from build123d import *

# Parameters (mm, degrees)
BOSS_EXTRUDE1_DEPTH = 2.5
SKETCH3_R           = 1
CUT_EXTRUDE1_DEPTH  = 5


with BuildPart() as part:
    # Sketch1 → Boss-Extrude1 (new, symmetric)
    with BuildSketch(Plane.XY):
        with BuildLine():
            ThreePointArc((-230.921678322, 34.636363636), (-231.800357978, 32.515043293), (-233.921678322, 31.636363636))
            Line((-233.921678322, 31.636363636), (-233.921678322, 29.636363636))
            ThreePointArc((-233.921678322, 29.636363636), (-233.356489225, 29.668410206), (-232.798545076, 29.764139123))
            ThreePointArc((-232.798545076, 29.764139123), (-230.009155719, 31.52313912), (-228.921678322, 34.636363636))
            Line((-228.921678322, 34.636363636), (-230.921678322, 34.636363636))
        make_face()
        with BuildLine():
            ThreePointArc((-233.921678322, 31.636363636), (-236.042998665, 32.515043293), (-236.921678322, 34.636363636))
            Line((-236.921678322, 34.636363636), (-238.921678322, 34.636363636))
            ThreePointArc((-238.921678322, 34.636363636), (-237.834200924, 31.52313912), (-235.044811567, 29.764139123))
            ThreePointArc((-235.044811567, 29.764139123), (-234.486867419, 29.668410206), (-233.921678322, 29.636363636))
            Line((-233.921678322, 29.636363636), (-233.921678322, 31.636363636))
        make_face()
        with BuildLine():
            ThreePointArc((-232.798545076, 29.764139123), (-233.356489225, 29.668410206), (-233.921678322, 29.636363636))
            Line((-233.921678322, 29.636363636), (-233.921678322, 28.764139123))
            Line((-233.921678322, 28.764139123), (-232.798545076, 28.764139123))
            Line((-232.798545076, 28.764139123), (-232.798545076, 29.764139123))
        make_face()
        with BuildLine():
            ThreePointArc((-233.921678322, 29.636363636), (-234.486867419, 29.668410206), (-235.044811567, 29.764139123))
            Line((-235.044811567, 29.764139123), (-235.044811567, 28.764139123))
            Line((-235.044811567, 28.764139123), (-233.921678322, 28.764139123))
            Line((-233.921678322, 28.764139123), (-233.921678322, 29.636363636))
        make_face()
    extrude(amount=BOSS_EXTRUDE1_DEPTH, both=True)

    # Sketch3 → Cut-Extrude1 (cut)
    with BuildSketch(Plane.XZ.offset(-28.764139123)):
        with Locations(Location((-233.921678322, 0, 0), (0, 0, 270))):
            Circle(SKETCH3_R)
    extrude(amount=-CUT_EXTRUDE1_DEPTH, mode=Mode.SUBTRACT)


solid = part.part
Check sheet for the modelled part. Datum: model origin and axes. Units: mm. Round coordinates to 2 decimals unless told otherwise and drop trailing zeros. Loops run counter-clockwise (first coordinate to the right, second up) from the corner with the lowest first, then second, coordinate; pieces in that order, holes last. Notation, with made-up numbers: (79, -2) -> (84, -2) arc R13 cw to (84, 22) -> close; hole circle Ø8 at (89.25, 44). An arc over 180 degrees is marked (long way). Put each result on its own line as item: value. Start each with the question number.
1. Scan lines: probe 1 along X at (y, z) = (29.1, 1.6); probe 2 along X at (y, z) = (32.1, -2.1); probe 3 along X at (y, z) = (34.45, -1.5). Record each from-to range of solid material in increasing order.
2. Section check C-C (z = 1.7). Enter the section's corners in (x, y).
3. Section check D-D (y = 33.9). Enter the section's corners in (x, z).
4. Section check A-A (z = 0). Enter the section's corners in (x, y), plus the area to 3 significant figures.
5. Draft check along X on faces 1 (the face through (-232.83, 31.84, -0.52)), 2 (the face through (-232.93, 30.27, 0.13)), 3 (the face through (-234, 31, 2.5)), 4 (the face through (-230.039, 31.486, 0.035)). Enter one of: +X half, -X half, draft (parallel to the pull), parting line (faces both ways), or undercut.
6. Section check B-B (y = 32.05). Enter the section's corners in (x, z).
7. Gauge pin test, flat ends, axial feed: pin 1 (1 mm diameter, centred on y = 33, z = -1.5, fed in from +X); pin 2 (1.1 mm diameter, centred on y = 29.5, z = 1, fed in from +X); pin 3 (1.5 mm diameter, centred on y = 32.5, z = -0.5, fed in from -X). Record the tip position at first contact, or that the pin passes through.
Findings:
1. probe 1: x = -235.04 to -232.8
1. probe 2: x = -238.23 to -235.52, -232.32 to -229.61
1. probe 3: x = -238.92 to -236.92, -230.93 to -228.93
2. outline: (-238.92, 34.64) arc R5 ccw to (-235.04, 29.76) -> (-235.04, 28.76) -> (-232.8, 28.76) -> (-232.8, 29.76) arc R5 ccw to (-228.92, 34.64) -> (-230.92, 34.64) arc R3 cw to (-236.92, 34.64) -> close
3. outline: (-238.87, -2.5) -> (-236.83, -2.5) -> (-236.83, 2.5) -> (-238.87, 2.5) -> close; (-231.01, -2.5) -> (-228.98, -2.5) -> (-228.98, 2.5) -> (-231.01, 2.5) -> close
4. outline: (-238.92, 34.64) arc R5 ccw to (-235.04, 29.76) -> (-235.04, 28.76) -> (-234.92, 28.76) -> (-234.92, 31.81) arc R3 cw to (-236.92, 34.64) -> close; (-232.92, 28.76) -> (-232.8, 28.76) -> (-232.8, 29.76) arc R5 ccw to (-228.92, 34.64) -> (-230.92, 34.64) arc R3 cw to (-232.92, 31.81) -> close
4. area: 21.3 mm^2
5. face 1: undercut
5. face 2: undercut
5. face 3: draft
5. face 4: +X half
6. outline: (-238.2, -2.5) -> (-235.44, -2.5) -> (-235.44, 2.5) -> (-238.2, 2.5) -> close; (-232.4, -2.5) -> (-229.64, -2.5) -> (-229.64, 2.5) -> (-232.4, 2.5) -> close
7. pin 1: stops at x = -229.05
7. pin 2: stops at x = -231.93
7. pin 3: stops at x = -238.73
